The model under review builds one solid part; all positions refer to its coordinate system, in mm. Face numbers are marked on the shaded views. Round coordinates to 2 decimals unless told otherwise and drop trailing zeros. Loops run counter-clockwise (first coordinate to the right, second up) from the corner with the lowest first, then second, coordinate; pieces in that order, holes last. Notation, with made-up numbers: (-3.75, -20.75) -> (22.25, -20.75) arc R25 cw to (22.25, 13.25) -> close; hole circle Ø6 at (-6, -20). An arc over 180 degrees is marked (long way). Use a Markdown table: item, result. Add a question column.
1) Wall thickness on probe 1 along Y at (x, z) = (6, 5); probe 2 along X at (y, z) = (-193.75, 5.25); probe 3 along Y at (x, z) = (6, 1): over which ranges is each line inside the solid? List them lowest first.
2) Insertion check: pin 1 (5.5 mm diameter, centred on x = 43.5, y = -2, fed in from +Z); pin 2 (1 mm diameter, centred on x = 27.5, z = 21, fed in from +Y); pin 3 (6.5 mm diameter, centred on y = -193.8, z = 43.4, fed in from -X); pin 4 (8 mm diameter, centred on y = -64, z = 36, fed in from -X). Each pin has a flat end and moves straight along its axis. Give the tip position at first contact, or say it passes through.
3) Consider section D-D on x = 53. Give the boundary of the cut face in (y, z).
4) Consider section C-C on y = -56. Give the boundary of the cut face in (x, z), plus the area to 3 significant figures.
5) Consider section B-B on z = 14.5. Give the boundary of the cut face in (x, y).
6) Consider section A-A on z = 43.4. Give the boundary of the cut face in (x, y).
7) Mouldability with a two-part tool opening along Z and no side actions: class the marked faces 1, 2, 3 and 4 as released by +Z, released by -Z, zero draft, split by the parting line, or undercut.
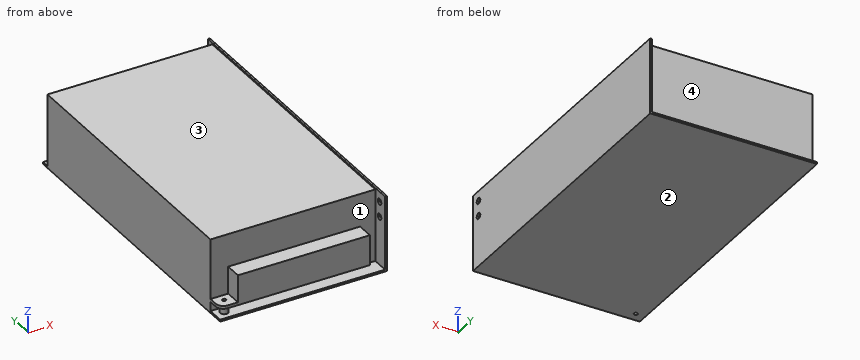
from build123d import *

# Parameters (mm, degrees)
F1_DEPTH  = 200
F2_W      = 108.7
F2_H      = 184
F3_DEPTH  = 47.7
F5_R      = 2.6
F5_R_2    = 1.25
F6_DEPTH  = 6.1
F7_R      = 2.6
F7_R_2    = 1.25
F8_DEPTH  = 1.9
F9_W      = 87
F9_H      = 11
F10_DEPTH = 18
F4_R      = 2
F11_DEPTH = 110.001
F12_DEPTH = 1.301


with BuildPart() as f1:
    # F0 (on Front) → F1 (new body)
    with BuildSketch(Plane.XZ):
        Polygon((0, 1.3), (0, 0), (110, 0), (110, 50), (108.7, 50), (108.7, 1.3), align=None)
    extrude(amount=F1_DEPTH)

    # F2 (on face) → F3 (join, through all)
    with BuildSketch(Plane.XY.offset(1.3)):
        with Locations((54.35, -97)):
            Rectangle(F2_W, F2_H)
    extrude(amount=F3_DEPTH)

    # F5 (on face) → F6 (join)
    with BuildSketch(Plane.XY.offset(1.3)):
        with Locations((6.25, -193.75)):
            Circle(F5_R)
        with Locations((6.25, -193.75)):
            Circle(F5_R_2, mode=Mode.SUBTRACT)
    extrude(amount=F6_DEPTH)

    # F7 (on face) → F8 (join)
    with BuildSketch(Plane.XY.offset(7.4)):
        with BuildLine():
            Line((98.7, -200), (98.7, -189))
            Line((98.7, -189), (0, -189))
            Line((0, -189), (0, -195))
            ThreePointArc((0, -195), (1.4644660941, -198.5355339059), (5, -200))
            Line((5, -200), (98.7, -200))
        make_face()
        with Locations((6.25, -193.75)):
            Circle(F7_R, mode=Mode.SUBTRACT)
        with Locations((6.25, -193.75)):
            Circle(F7_R)
        with Locations((6.25, -193.75)):
            Circle(F7_R_2, mode=Mode.SUBTRACT)
    extrude(amount=F8_DEPTH)

    # F9 (on face) → F10 (join)
    with BuildSketch(Plane.XY.offset(9.3)):
        with Locations((55.2, -194.5)):
            Rectangle(F9_W, F9_H)
    extrude(amount=F10_DEPTH)

    # F4 (on face) → F11 (cut, through all)
    with BuildSketch(Plane.YZ.offset(110)):
        with Locations((-193.8, 43.4)):
            Circle(F4_R)
        with Locations((-193.8, 33.4)):
            Circle(F4_R)
    extrude(amount=-F11_DEPTH, mode=Mode.SUBTRACT)

    # F12 (cut, through all): a face of the model
    f12_faces = [f1.faces().sort_by_distance(p)[0] for p in [
        (6.25, -193.75, 1.3),
    ]]
    extrude(f12_faces, amount=-F12_DEPTH, mode=Mode.SUBTRACT)


solid = f1.part
Result set:
| question | item | result |
|---|---|---|
| 1 | probe 1 | -196.34 to -194.97, -192.53 to -191.16, -189 to -5 |
| 1 | probe 2 | 3.65 to 5, 7.5 to 8.85, 108.7 to 110 |
| 1 | probe 3 | -200 to -194.97, -192.53 to 0 |
| 2 | pin 1 | z = 1.3 |
| 2 | pin 2 | y = -5 |
| 2 | pin 3 | x = 108.7 |
| 2 | pin 4 | x = 0 |
| 3 | outline | (-200, 0) -> (0, 0) -> (0, 1.3) -> (-5, 1.3) -> (-5, 49) -> (-189, 49) -> (-189, 27.3) -> (-200, 27.3) -> (-200, 7.4) -> (-189, 7.4) -> (-189, 1.3) -> (-200, 1.3) -> close |
| 4 | outline | (0, 0) -> (110, 0) -> (110, 50) -> (108.7, 50) -> (108.7, 49) -> (0, 49) -> close |
| 4 | area | 5,390 mm2 |
| 5 | outline | (0, -189) -> (11.7, -189) -> (11.7, -200) -> (98.7, -200) -> (98.7, -189) -> (108.7, -189) -> (108.7, -200) -> (110, -200) -> (110, 0) -> (108.7, 0) -> (108.7, -5) -> (0, -5) -> close |
| 6 | outline | (0, -189) -> (108.7, -189) -> (108.7, -191.8) -> (110, -191.8) -> (110, 0) -> (108.7, 0) -> (108.7, -5) -> (0, -5) -> close; (108.7, -200) -> (110, -200) -> (110, -195.8) -> (108.7, -195.8) -> close |
| 7 | face 1 | undercut |
| 7 | face 2 | released by -Z |
| 7 | face 3 | released by +Z |
| 7 | face 4 | zero draft |
